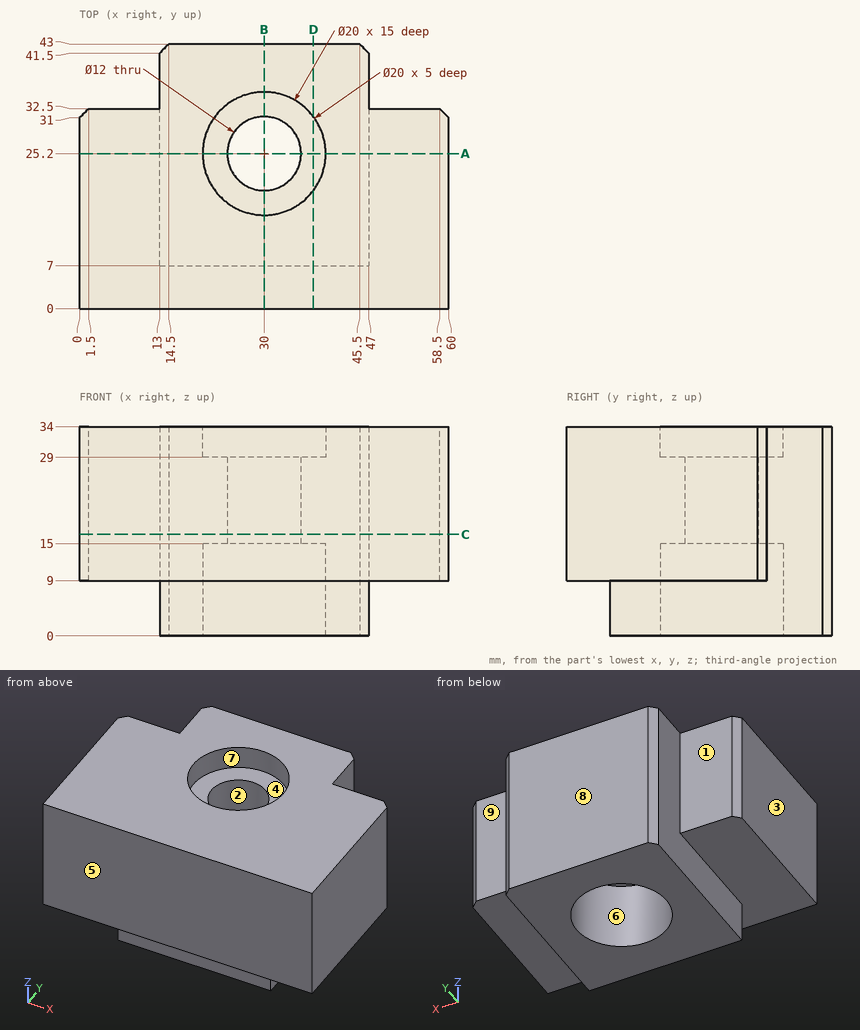
Geometry check sheet. Reference: drawing and pictorial views, mm from the part's lowest x, y, z. A direction names the side the tool comes from. Round coordinates to 2 decimals unless told otherwise and drop trailing zeros. Write each loop counter-clockwise with the first axis right and the second up, starting at its lowest first coordinate (ties: lowest second). Pieces come first, ordered by that corner, then holes.
(1) Depth check by flat-ended pin: pin 1 Ø16 at (x, y) = (30, 25.2) entering from +Z; pin 2 Ø10 at (x, z) = (53.5, 17.5) entering from +Y; pin 3 Ø4.5 at (x, z) = (26, 4) entering from -Y. Enter the tip coordinate at first touch or a pass-through.
Returned:
pin 1: stops at z = 29
pin 2: stops at y = 32.5
pin 3: stops at y = 7
(2) Section check C-C (z = 16.5). Enter the section's corners in (x, y), plus the area to 3 significant figures.
Returned:
outline: (0, 0) - (60, 0) - (60, 31) - (58.5, 32.5) - (47, 32.5) - (47, 41.5) - (45.5, 43) - (14.5, 43) - (13, 41.5) - (13, 32.5) - (1.5, 32.5) - (0, 31) - close; hole circle Ø12 at (30, 25.2)
area: 2,190 mm2
(3) Mould release check, pull along X, two halves, no side actions. Record for the marked faces 1, 2, 3 and 4: pulls with the +X half, pulls with the -X half, needs draft (parallel to the pull), parting line crosses it, or undercut.
Returned:
face 1: needs draft
face 2: undercut
face 3: pulls with the -X half
face 4: undercut
(4) Section check D-D (x = 38). Enter the section's corners in (y, z), plus the area to 3 significant figures.
Returned:
outline: (0, 9) - (7, 9) - (7, 0) - (19.2, 0) - (19.2, 15) - (31.2, 15) - (31.2, 0) - (43, 0) - (43, 34) - (31.2, 34) - (31.2, 29) - (19.2, 29) - (19.2, 34) - (0, 34) - close
area: 1,160 mm2
(5) Section check B-B (x = 30). Enter the section's corners in (y, z).
Returned:
outline: (0, 9) - (7, 9) - (7, 0) - (15.2, 0) - (15.2, 15) - (19.2, 15) - (19.2, 29) - (15.2, 29) - (15.2, 34) - (0, 34) - close; (31.2, 15) - (35.2, 15) - (35.2, 0) - (43, 0) - (43, 34) - (35.2, 34) - (35.2, 29) - (31.2, 29) - close
(6) Access from +Z, -Z, +X, -X, +Y, -Y to the whole of each face (thin tool, end or side, straight path). Record for the marked faces 5, 6, 7, 8 and 9.
Returned:
face 5: +Z, -Z, +X, -X, -Y
face 6: -Z
face 7: +Z
face 8: +Z, -Z, +X, -X, +Y
face 9: +Z, -Z, +X, +Y
(7) Material ranges on line 1 (Y direction, x = 30, z = 31.6); line 2 (Y direction, x = 30, z = 5); line 3 (X direction, y = 25, z = 11), recorded low to high.
Returned:
line 1: y = 0 to 15.2, 35.2 to 43
line 2: y = 7 to 15.2, 35.2 to 43
line 3: x = 0 to 20, 40 to 60
(8) Section check A-A (y = 25.2). Enter the section's corners in (x, z).
Returned:
outline: (0, 9) - (13, 9) - (13, 0) - (20, 0) - (20, 15) - (24, 15) - (24, 29) - (20, 29) - (20, 34) - (0, 34) - close; (36, 15) - (40, 15) - (40, 0) - (47, 0) - (47, 9) - (60, 9) - (60, 34) - (40, 34) - (40, 29) - (36, 29) - close
